from build123d import *

# Parameters (mm, degrees)
BOSS_EXTRUDE1_DEPTH = 10
FILLET3_R           = 3
CUT_EXTRUDE8_START  = -33
SKETCH8_R           = 2
CUT_EXTRUDE8_DEPTH  = 197.665485806
SKETCH11_R          = 3
CUT_EXTRUDE9_DEPTH  = 35
SKETCH7_W           = 2
SKETCH7_H           = 30
CUT_EXTRUDE10_DEPTH = 5
CUT_EXTRUDE11_DEPTH = 5
CUT_EXTRUDE12_DEPTH = 5
CIRPATTERN8_COUNT   = 3
SKETCH17_W          = 14
SKETCH17_H          = 4
BOSS_EXTRUDE3_DEPTH = 3
CIRPATTERN9_COUNT   = 3


with BuildPart() as part:
    # Sketch2 → Boss-Extrude1 (new body)
    with BuildSketch(Plane(origin=(0, 0, 0), x_dir=(1, 0, 0), z_dir=(0, 1, 0))):
        Polygon((10, 5.773502692), (10, 70), (-10, 70), (-10, 5.773502692), (-65.621778265, -26.339745962), (-55.621778265, -43.660254038), (0, -11.547005384), (55.621778265, -43.660254038), (65.621778265, -26.339745962), align=None)
    extrude(amount=BOSS_EXTRUDE1_DEPTH)

    # Fillet3
    fillet3_edges = [part.edges().sort_by_distance(p)[0] for p in [
        (-37.810889132, 10, 10.283121635),
        (-27.810889132, 0, 27.603629711),
        (-60.621778265, 0, 35),
        (-37.810889132, 0, 10.283121635),
        (-10, 0, -37.886751346),
        (0, 0, -70),
        (-60.621778265, 10, 35),
        (10, 5, -70),
        (10, 5, -5.773502692),
        (65.621778265, 5, 26.339745962),
        (55.621778265, 5, 43.660254038),
        (0, 5, 11.547005384),
        (-55.621778265, 5, 43.660254038),
        (-65.621778265, 5, 26.339745962),
        (-10, 5, -5.773502692),
        (-10, 5, -70),
        (-27.810889132, 10, 27.603629711),
        (27.810889132, 10, 27.603629711),
        (60.621778265, 10, 35),
        (37.810889132, 10, 10.283121635),
        (10, 10, -37.886751346),
        (0, 10, -70),
        (-10, 10, -37.886751346),
        (10, 0, -37.886751346),
        (37.810889132, 0, 10.283121635),
        (60.621778265, 0, 35),
        (27.810889132, 0, 27.603629711),
    ]]
    fillet(fillet3_edges, radius=FILLET3_R)

    # Sketch8 → Cut-Extrude8 (cut)
    with BuildSketch(Plane(origin=(60.621778265, 0, 35), x_dir=(0.49999999999999983, 0, -0.8660254037844388), z_dir=(0.8660254037844387, 0, 0.4999999999999998)).offset(CUT_EXTRUDE8_START)):
        with Locations(Location((0, 5, 0), (0, 0, 90))):
            Circle(SKETCH8_R)
    cut_extrude8 = extrude(amount=CUT_EXTRUDE8_DEPTH, mode=Mode.SUBTRACT)

    # Sketch11 → Cut-Extrude9 (cut)
    with BuildSketch(Plane(origin=(32.04293994, 0, 18.5), x_dir=(0.49999999999999994, 0, -0.8660254037844387), z_dir=(0.8660254037844386, 0, 0.4999999999999999))):
        with Locations((0, 5)):
            Circle(SKETCH11_R)
    cut_extrude9 = extrude(amount=-CUT_EXTRUDE9_DEPTH, mode=Mode.SUBTRACT)

    # Sketch7 → Cut-Extrude10 (cut)
    with BuildSketch(Plane(origin=(0, 10, 0), x_dir=(1, 0, 0), z_dir=(0, 1, 0))):
        with Locations((0.025333085, 52)):
            Rectangle(SKETCH7_W, SKETCH7_H)
    extrude(amount=-CUT_EXTRUDE10_DEPTH, mode=Mode.SUBTRACT)

    # Sketch7_7 → Cut-Extrude11 (cut)
    with BuildSketch(Plane(origin=(0, 10, 0), x_dir=(1, 0, 0), z_dir=(0, 1, 0))):
        Polygon((-58.536368596, -32.612035501), (-32.555606483, -17.612035501), (-31.555606483, -19.344086308), (-57.536368596, -34.344086308), align=None)
    extrude(amount=-CUT_EXTRUDE11_DEPTH, mode=Mode.SUBTRACT)

    # Sketch7_8 → Cut-Extrude12 (cut)
    with BuildSketch(Plane(origin=(0, 10, 0), x_dir=(1, 0, 0), z_dir=(0, 1, 0))):
        Polygon((31.530273397, -19.387964499), (57.511035511, -34.387964499), (58.511035511, -32.655913692), (32.530273397, -17.655913692), align=None)
    extrude(amount=-CUT_EXTRUDE12_DEPTH, mode=Mode.SUBTRACT)

    # CirPattern8: Cut-Extrude8, Cut-Extrude9 ×3 about axis
    cirpattern8_axis = Axis((0, 0, 0), (0, 1, 0))
    add([cut_extrude8.rotate(cirpattern8_axis, i * 360 / CIRPATTERN8_COUNT) for i in range(1, CIRPATTERN8_COUNT)], mode=Mode.SUBTRACT)
    add([cut_extrude9.rotate(cirpattern8_axis, i * 360 / CIRPATTERN8_COUNT) for i in range(1, CIRPATTERN8_COUNT)], mode=Mode.SUBTRACT)

    # Sketch17 → Boss-Extrude3 (add)
    with BuildSketch(Plane(origin=(60.621778265, 0, 35), x_dir=(0.49999999999999983, 0, -0.8660254037844388), z_dir=(0.8660254037844387, 0, 0.4999999999999998))):
        with Locations((0, 5)):
            Rectangle(SKETCH17_W, SKETCH17_H)
    boss_extrude3 = extrude(amount=-BOSS_EXTRUDE3_DEPTH)

    # CirPattern9: Boss-Extrude3 ×3 about axis
    cirpattern9_axis = Axis((0, 10, 0), (0, 1, 0))
    for i in range(1, CIRPATTERN9_COUNT):
        add(boss_extrude3.rotate(cirpattern9_axis, i * 360 / CIRPATTERN9_COUNT))


solid = part.part
Verification items for the finished model (mm, model axes). A direction names the side the tool comes from. Coordinates: 2 decimals unless noted, no trailing zeros. Write each loop counter-clockwise with the first axis right and the second up, starting at its lowest first coordinate (ties: lowest second). Pieces come first, ordered by that corner, then holes. Notation, with made-up numbers: (66, -14.5) -> (74, -14.5) arc R20 cw to (74, 15.5) -> close; hole circle Ø7 at (7.5, 1). An arc over 180 degrees is marked (long way). One line per item, written item: value. Start each with the question number.
Q1. Thickness scan on L1, parallel to X at y = 5, z = -14; L2, parallel to X at y = 6, z = 7; L3, parallel to X at y = 7.25, z = 0. Record the ranges inside material, lowest first. Write a range as from..to.
Q2. Mould release check, pull along Y, two halves, no side actions. Record for faces 1 (the cylindrical face through (-37.195, 9.098, 10.915)), 2 (the flat face through (-1, 3, -37)), 3 (the flat face through (45.7, 8.4, 25.26)): pulls with the +Y half, pulls with the -Y half, needs draft (parallel to the pull), parting line crosses it, or undercut.
Q3. Go/stop test with flat-tipped pins: P1, Ø1, axis at y = 7.5, z = -47, coming from the +X side; P2, Ø6, axis at x = -23, y = 8, coming from the +Z side; P3, Ø3, axis at y = 5.5, z = -30.5, coming from the -X side. Record where each tip stops, or that it passes through.
Q4. Cross-section at B-B on z = -44. Enter the section's corners in (x, y), and give its area (3 significant figures).
Q5. Cross-section at A-A on z = -28.5. Enter the section's corners in (x, y).
Q6. Cross-section at C-C on y = 5. State how many separate pieces and enclosed holes the cut face has, and give its area (3 significant figures).
Q7. Access from +Z, -Z, +X, -X, +Y, -Y to the whole of each face (thin tool, end or side, straight path). Record for faces 4 (the cylindrical face through (28.05, 9.1, 26.75)), 5 (the flat face through (0, 7, -67)), 6 (the cylindrical face through (-27.329, 0.902, 26.338)).
Checked values:
1. L1: x = -10..-3, 3..10
1. L2: x = -32.12..-17.78, -6.47..6.47, 17.78..32.12
1. L3: x = -19.98..-3.97, -2.31..2.31, 3.97..19.98
2. face 1: pulls with the +Y half
2. face 2: undercut
2. face 3: needs draft
3. P1: stops at x = 10
3. P2: stops at z = 26.49
3. P3: stops at x = -10
4. outline: (-10, 3) arc R3 ccw to (-7, 0) -> (7, 0) arc R3 ccw to (10, 3) -> (10, 7) arc R3 ccw to (7, 10) -> (1.03, 10) -> (1.03, 6.72) arc R2 cw (long way) to (-0.97, 6.75) -> (-0.97, 10) -> (-7, 10) arc R3 ccw to (-10, 7) -> close
4. area: 174 mm²
5. outline: (-10, 3) arc R3 ccw to (-7, 0) -> (7, 0) arc R3 ccw to (10, 3) -> (10, 7) arc R3 ccw to (7, 10) -> (-7, 10) arc R3 ccw to (-10, 7) -> close; hole circle Ø6 at (0, 5)
6. separate pieces: 1
6. enclosed holes: 3
6. area: 3,030 mm²
7. face 4: +Z, +Y
7. face 5: none
7. face 6: +Z, -Y
